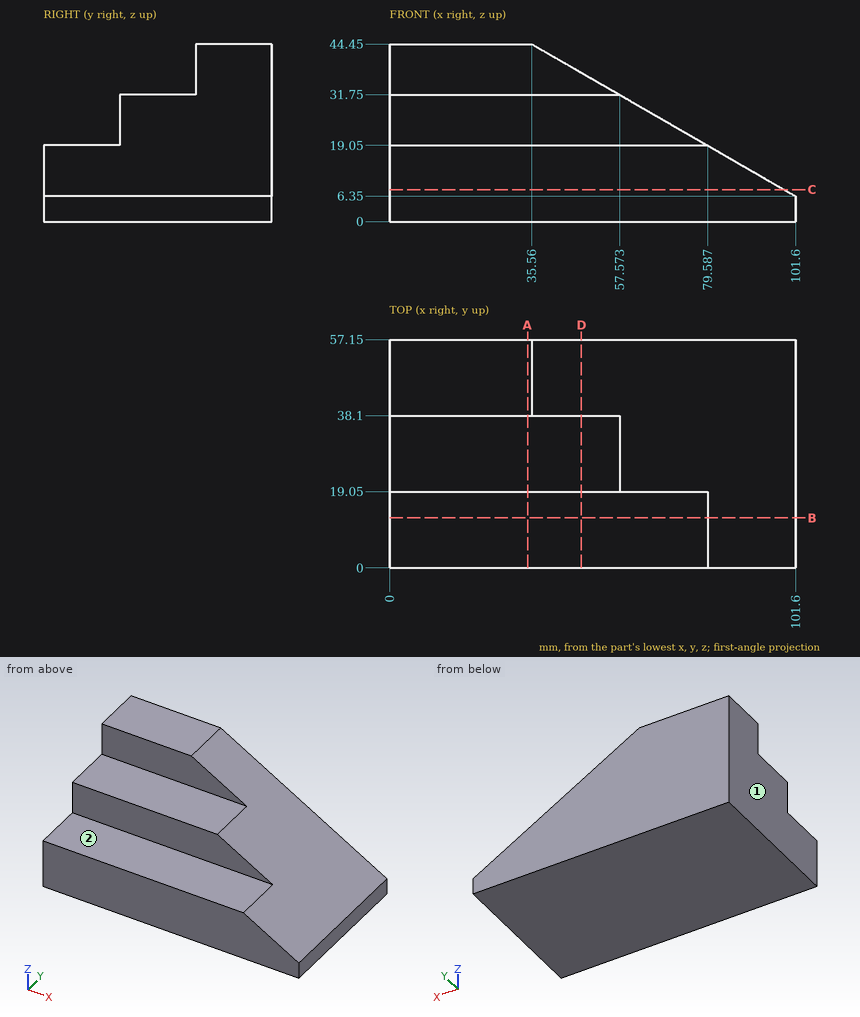
Here's the drawing with two shaded views (mm, measured from the low corner). I have some questions. A direction names the side the tool comes from. Coordinates: 2 decimals unless noted, no trailing zeros. Write each loop counter-clockwise with the first axis right and the second up, starting at its lowest first coordinate (ties: lowest second). Pieces come first, ordered by that corner, then holes. Notation, with made-up numbers: (84.5, 64) -> (134.5, 64) arc R20 ccw to (134.5, 95) -> close; hole circle Ø6 at (24, 43.25). An arc over 180 degrees is marked (long way). Use a Markdown table: item, result. Add a question column.
(1) If we section it at C-C, the plane z = 8: Write out the boundary of the cut face in (x, y), and give its area (3 significant figures).
(2) For the marked faces 1 and 2, which set-ups out of +Z, -Z, +X, -X, +Y, -Y let a thin tool reach every point of the face, with its end or its side?
(3) If we section it at A-A, the plane x = 34.5: Write out the boundary of the cut face in (y, z), and give its area (3 significant figures).
(4) If we section it at B-B, the plane y = 12.5: Write out the boundary of the cut face in (x, z), and give its area (3 significant figures).
(5) If we section it at D-D, the plane x = 48: Write out the boundary of the cut face in (y, z).
(6) I'm going to push flat-ended pins straight in: P1, Ø3, axis at y = 49.5, z = 37.5, coming from the +X side (1 decimal); P2, Ø3, axis at y = 42.5, z = 30.5, coming from the +X side; P3, Ø21, axis at x = 23.5, y = 26.5, coming from the +Z side. Where does each tip first touch, or does it pass through?
(7) Please list where these lines run through material, in increasing order: line 1 (Z direction, x = 26, y = 27.5); line 2 (Z direction, x = 44, y = 9.5); line 3 (X direction, y = 50.5, z = 23.5) (1 decimal).
Outcome:
| question | item | result |
|---|---|---|
| 1 | outline | (0, 0) -> (98.74, 0) -> (98.74, 57.15) -> (0, 57.15) -> close |
| 1 | area | 5,640 mm^2 |
| 2 | face 1 | +Z, -Z, -X, +Y, -Y |
| 2 | face 2 | +Z, +X, -X, -Y |
| 3 | outline | (0, 0) -> (57.15, 0) -> (57.15, 44.45) -> (38.1, 44.45) -> (38.1, 31.75) -> (19.05, 31.75) -> (19.05, 19.05) -> (0, 19.05) -> close |
| 3 | area | 1,810 mm^2 |
| 4 | outline | (0, 0) -> (101.6, 0) -> (101.6, 6.35) -> (79.59, 19.05) -> (0, 19.05) -> close |
| 4 | area | 1,800 mm^2 |
| 5 | outline | (0, 0) -> (57.15, 0) -> (57.15, 37.27) -> (38.1, 37.27) -> (38.1, 31.75) -> (19.05, 31.75) -> (19.05, 19.05) -> (0, 19.05) -> close |
| 6 | P1 | stops at x = 50.2 |
| 6 | P2 | stops at x = 62.34 |
| 6 | P3 | stops at z = 31.75 |
| 7 | line 1 | z = 0 to 31.75 |
| 7 | line 2 | z = 0 to 19.05 |
| 7 | line 3 | x = 0 to 71.9 |
